Design review of the part built by this model. Coordinates are the model's own, in mm. Face numbers are marked on the shaded views. Coordinates: 2 decimals unless noted, no trailing zeros. Write each loop counter-clockwise with the first axis right and the second up, starting at its lowest first coordinate (ties: lowest second). Pieces come first, ordered by that corner, then holes.
Q1. For probe 1 along X at (y, z) = (-1.25, 2.7); probe 2 along Y at (x, z) = (7.25, 3.1); probe 3 along Y at (x, z) = (4.5, 0.45), list the stretches that pass through material, from the lowest coordinate up.
Q2. Take a section at C-C (y = -0.75). Give the boundary of the cut face in (x, z).
Q3. Take a section at D-D (x = -11.5). Give the boundary of the cut face in (y, z), and give its area (3 significant figures).
Q4. Insertion check: pin 1 (1 mm diameter, centred on y = -4.5, z = 2.5, fed in from -X); pin 2 (0.8 mm diameter, centred on x = 0, y = -0.5, fed in from +Z); pin 3 (2 mm diameter, centred on x = 0, y = 0, fed in from -Z). Each pin has a flat end and moves straight along its axis. Give the tip position at first contact, or say it passes through.
Q5. Take a section at A-A (z = 2.35). Give the boundary of the cut face in (x, y), and give its area (3 significant figures).
Q6. Take a section at B-B (x = 1). Give the boundary of the cut face in (y, z).
Q7. Mouldability with a two-part tool opening along X and no side actions: class the marked faces 1, 2, 3 and 4 as pulls with the +X half, pulls with the -X half, needs draft (parallel to the pull), parting line crosses it, or undercut.
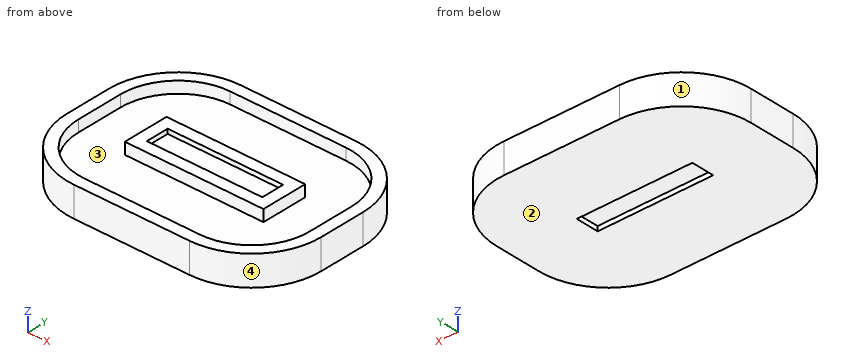
```python
from build123d import *

# Parameters (mm, degrees)
F0_W     = 12.7
F0_H     = 2.54
F1_DEPTH = 3.302
F2_W     = 15.24
F2_H     = 5.08
F3_DEPTH = 1.27
F2_W_2   = 12.7
F2_H_2   = 2.54
F4_DEPTH = 0.508
F5_DEPTH = 0.508


with BuildPart() as f1:
    # F0 (on Top) → F1 (new body)
    with BuildSketch(Plane.XY):
        with BuildLine():
            Line((-6.35, -10.16), (6.35, -10.16))
            ThreePointArc((6.35, -10.16), (11.738154, -7.928154), (13.97, -2.54))
            Line((13.97, -2.54), (13.97, 2.54))
            ThreePointArc((13.97, 2.54), (11.738154, 7.928154), (6.35, 10.16))
            Line((6.35, 10.16), (-6.35, 10.16))
            ThreePointArc((-6.35, 10.16), (-11.738154, 7.928154), (-13.97, 2.54))
            Line((-13.97, 2.54), (-13.97, -2.54))
            ThreePointArc((-13.97, -2.54), (-11.738154, -7.928154), (-6.35, -10.16))
        make_face()
        Rectangle(F0_W, F0_H, mode=Mode.SUBTRACT)
        Rectangle(F0_W, F0_H)
    extrude(amount=F1_DEPTH)

    # F2 (on face) → F3 (cut)
    with BuildSketch(Plane.XY.offset(3.302)):
        with BuildLine():
            Line((-6.35, -8.89), (6.35, -8.89))
            ThreePointArc((6.35, -8.89), (10.840128, -7.030128), (12.7, -2.54))
            Line((12.7, -2.54), (12.7, 2.54))
            ThreePointArc((12.7, 2.54), (10.840128, 7.030128), (6.35, 8.89))
            Line((6.35, 8.89), (-6.35, 8.89))
            ThreePointArc((-6.35, 8.89), (-10.840128, 7.030128), (-12.7, 2.54))
            Line((-12.7, 2.54), (-12.7, -2.54))
            ThreePointArc((-12.7, -2.54), (-10.840128, -7.030128), (-6.35, -8.89))
        make_face()
        Rectangle(F2_W, F2_H, mode=Mode.SUBTRACT)
    extrude(amount=-F3_DEPTH, mode=Mode.SUBTRACT)

    # F2 (on face) → F4 (cut)
    with BuildSketch(Plane.XY.offset(3.302)):
        Rectangle(F2_W_2, F2_H_2)
    extrude(amount=-F4_DEPTH, mode=Mode.SUBTRACT)

    # F0 (on Top) → F5 (cut)
    with BuildSketch(Plane.XY):
        Rectangle(F0_W, F0_H)
    extrude(amount=F5_DEPTH, mode=Mode.SUBTRACT)


solid = f1.part
```
Response:
1. probe 1: x = -13.97 to -12.7, -7.62 to 7.62, 12.7 to 13.97
1. probe 2: y = -10.11 to -8.83, -2.54 to 2.54, 8.83 to 10.11
1. probe 3: y = -10.16 to -1.27, 1.27 to 10.16
2. outline: (-13.97, 0) - (-6.35, 0) - (-6.35, 0.51) - (6.35, 0.51) - (6.35, 0) - (13.97, 0) - (13.97, 3.3) - (12.7, 3.3) - (12.7, 2.03) - (7.62, 2.03) - (7.62, 3.3) - (6.35, 3.3) - (6.35, 2.79) - (-6.35, 2.79) - (-6.35, 3.3) - (-7.62, 3.3) - (-7.62, 2.03) - (-12.7, 2.03) - (-12.7, 3.3) - (-13.97, 3.3) - close
3. outline: (-8.16, 0) - (8.16, 0) - (8.16, 3.3) - (6.25, 3.3) - (6.25, 2.03) - (-6.25, 2.03) - (-6.25, 3.3) - (-8.16, 3.3) - close
3. area: 38.0 mm2
4. pin 1: stops at x = -13.83
4. pin 2: stops at z = 2.79
4. pin 3: stops at z = 0.51
5. outline: (-13.97, -2.54) arc R7.62 ccw to (-6.35, -10.16) - (6.35, -10.16) arc R7.62 ccw to (13.97, -2.54) - (13.97, 2.54) arc R7.62 ccw to (6.35, 10.16) - (-6.35, 10.16) arc R7.62 ccw to (-13.97, 2.54) - close; (-7.62, -2.54) - (7.62, -2.54) - (7.62, 2.54) - (-7.62, 2.54) - close; hole (-12.7, -2.54) arc R6.35 ccw to (-6.35, -8.89) - (6.35, -8.89) arc R6.35 ccw to (12.7, -2.54) - (12.7, 2.54) arc R6.35 ccw to (6.35, 8.89) - (-6.35, 8.89) arc R6.35 ccw to (-12.7, 2.54) - close
5. area: 178 mm2
6. outline: (-10.16, 0) - (-1.27, 0) - (-1.27, 0.51) - (1.27, 0.51) - (1.27, 0) - (10.16, 0) - (10.16, 3.3) - (8.89, 3.3) - (8.89, 2.03) - (2.54, 2.03) - (2.54, 3.3) - (1.27, 3.3) - (1.27, 2.79) - (-1.27, 2.79) - (-1.27, 3.3) - (-2.54, 3.3) - (-2.54, 2.03) - (-8.89, 2.03) - (-8.89, 3.3) - (-10.16, 3.3) - close
7. face 1: pulls with the -X half
7. face 2: needs draft
7. face 3: undercut
7. face 4: pulls with the +X half
